Source: CAD feature listing. Evaluate the final solid. Frame: model axes, mm. A direction names the side the tool comes from. Coordinates: 2 decimals unless noted, no trailing zeros. Loops run counter-clockwise (first coordinate to the right, second up) from the corner with the lowest first, then second, coordinate; pieces in that order, holes last.
Item 1: Section query B-B, the plane y = 17.5. Return the cut outline in (x, z) (3 decimals).
Item 2: Reachability of faces 1 (the flat face through (13, 22.225, -313)), 2 (the flat face through (13, 0, -313)) from +Z, -Z, +X, -X, +Y, -Y: full face, straight path, thin tool, end or side. Return the list, or none.
Item 3: Pull-direction query (X, two-part tool) for faces 3 (the flat face through (22.225, 13, -313)), 4 (the flat face through (13, 3.175, -313)), 5 (the flat face through (25.4, 13, -313)), 6 (the flat face through (13, 25.4, -313)); classes: +X half, -X half, draft (parallel to the pull), parting line (faces both ways), or undercut.
Item 4: Line query: probe 1 along Z at (x, y) = (12.7, 1.2) (3 decimals); probe 2 along X at (y, z) = (2.25, -12.7) (3 decimals); probe 3 along X at (y, z) = (10.25, -396.5) (3 decimals). Output: solid intervals per line, ascending.
Item 5: Section query A-A, the plane z = -149. Return the cut outline in (x, y) (3 decimals).
Item 6: Pin query (flat end, axial travel): pin 1 Ø2 at (y, z) = (22, -265) entering from -X. Return the tip coordinate at first contact, or that it passes through.
Autodesk Inventor part; units mm, degrees
ref_plane "YZ Plane" through (0, 0, 0) normal (1, 0, 0) x (0, 1, 0)
ref_plane "XZ Plane" through (0, 0, 0) normal (0, 1, 0) x (-1, 0, 0)
ref_plane "XY Plane" through (0, 0, 0) normal (0, 0, 1) x (1, 0, 0)
sketch "Sketch1" plane through (0, 0, 0) normal (0, 0, 1) x (1, 0, 0)
  line L0 (0, 0) -> (25.4, 0)
  line L1 (25.4, 0) -> (25.4, 25.4)
  line L2 (25.4, 25.4) -> (0, 25.4)
  line L3 (0, 25.4) -> (0, 0)
  line L4 (3.175, 22.225) -> (22.225, 22.225)
  line L5 (22.225, 22.225) -> (22.225, 3.175)
  line L6 (22.225, 3.175) -> (3.175, 3.175)
  line L7 (3.175, 3.175) -> (3.175, 22.225)
  dimension "d0" = 25.4
  dimension "d1" = 25.4
  dimension "d2" = 3.175
extrude "Extrusion1" add sketch "Sketch1" against normal blind 635
sketch "Sketch2" plane through (0, 25.4, 0) normal (0, 1, 0) x (1, 0, 0)
  line L0 (25.4, 0) -> (0, 0)
  point P0 (12.7, 12.7)
  point P1 (12.7, 38.1)
  dimension "d5" = 12.7
  dimension "d6" = 25.4
hole "Hole1" at (12.7, 25.4, -12.7) at (12.7, 25.4, -38.1) direction (0, -1, 0) diameter 6.35 depth 25.4 tip angle 118
properties part number "tophalf tallthing"
Verdict:
1. outline: (0, -635) - (3.175, -635) - (3.175, 0) - (0, 0) - close; (22.225, -635) - (25.4, -635) - (25.4, 0) - (22.225, 0) - close
2. face 1: +Z, -Z
2. face 2: +Z, -Z, +X, -X, -Y
3. face 3: undercut
3. face 4: undercut
3. face 5: +X half
3. face 6: draft
4. probe 1: z = -635 to -41.275, -34.925 to -15.875, -9.525 to 0
4. probe 2: x = 0 to 9.525, 15.875 to 25.4
4. probe 3: x = 0 to 3.175, 22.225 to 25.4
5. outline: (0, 0) - (25.4, 0) - (25.4, 25.4) - (0, 25.4) - close; hole (3.175, 3.175) - (22.225, 3.175) - (22.225, 22.225) - (3.175, 22.225) - close
6. pin 1: stops at x = 0
